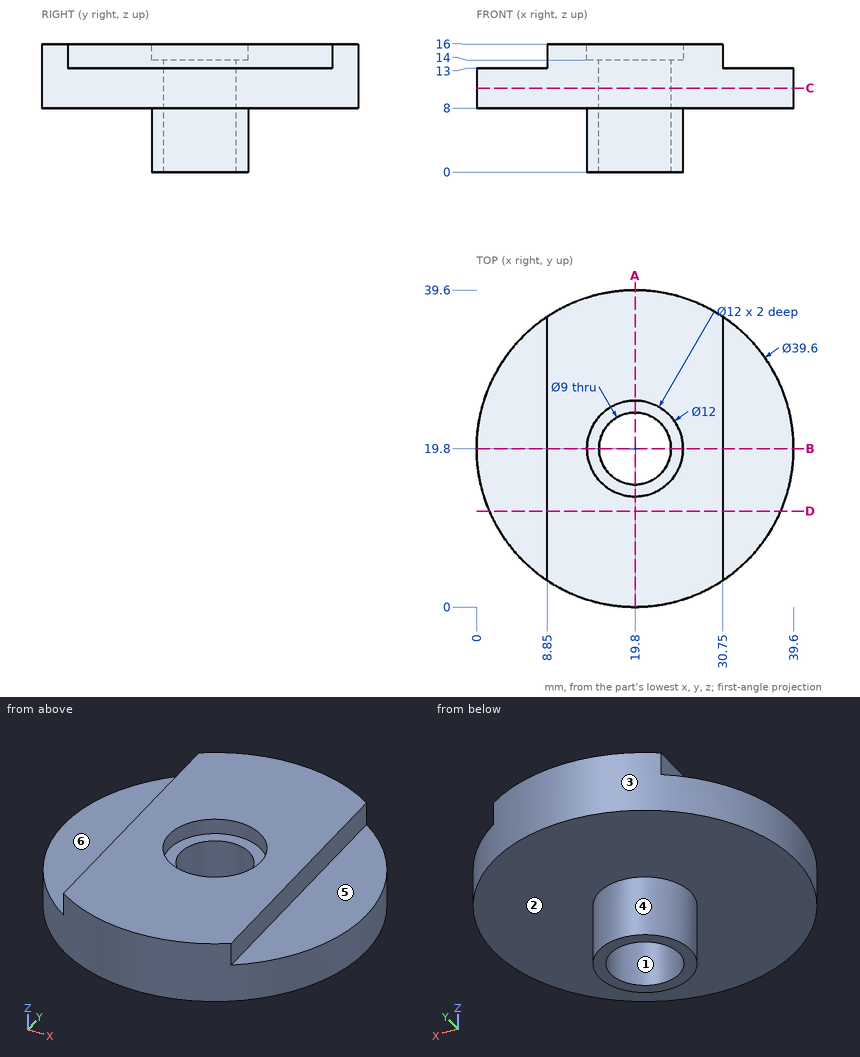
Could you check a few things on this drawing? It's one solid part, dimensions in mm from its lowest x, y, z. A direction names the side the tool comes from. Give positions to 0.01 mm unless a question says otherwise; leave off trailing zeros. Write each loop counter-clockwise with the first axis right and the second up, starting at its lowest first coordinate (ties: lowest second). Pieces come first, ordered by that corner, then holes. Notation, with made-up numbers: M 15.25,7 L 39.25,7 A8 cw 39.25,21 Z; hole C 38,37.5 d6. An arc over 180 degrees is marked long. Put each result on its own line as item: value. Start each with the question number.
Item 1: Will these pins go through, and if not, where does the flat tip stop? pin 1 (6 mm diameter, centred on y = 6, z = 7.5, fed in from -X); pin 2 (1.5 mm diameter, centred on y = 13.5, z = 14.5, fed in from -X); pin 3 (2 mm diameter, centred on y = 33, z = 10.5, fed in from +X).
Item 2: I need wall thicknesses on L1, parallel to X at y = 19.8, z = 6.75; L2, parallel to Y at x = 19.8, z = 10.75. Which ranges of each line are inside material? Lowest first, please. Write a range as from..to.
Item 3: Thinking about a two-plate mould opening in X: for the marked faces 1, 2 and 3, which applies, +X half, -X half, draft (parallel to the pull), parting line (faces both ways), or undercut?
Item 4: If we section it at D-D, the plane y = 12: Write out the boundary of the cut face in (x, z).
Item 5: If we section it at C-C, the plane z = 10.5: Write out the boundary of the cut face in (x, y), then the cut area to 3 significant figures.
Item 6: If we section it at A-A, the plane x = 19.8: Write out the boundary of the cut face in (y, z).
Item 7: If we section it at B-B, the plane y = 19.8: Write out the boundary of the cut face in (x, z), then the cut area to 3 significant figures.
Item 8: On a 3-axis mill with a long thin cutter (end or side, diameter ignored), from which of +Z, -Z, +X, -X, +Y, -Y can I reach the whole of each face in a straight line? I mean the marked faces 4, 5 and 6. Say none if no direction works.
Values:
1. pin 1: x = 3.23
1. pin 2: x = 8.85
1. pin 3: x = 35.39
2. L1: 13.8..15.3, 24.3..25.8
2. L2: 0..15.3, 24.3..39.6
3. face 1: undercut
3. face 2: draft
3. face 3: parting line
4. outline: M 1.6,8 L 38,8 L 38,13 L 30.75,13 L 30.75,16 L 8.85,16 L 8.85,13 L 1.6,13 Z
5. outline: C 19.8,19.8 d39.6; hole C 19.8,19.8 d9
5. area: 1,170 mm²
6. outline: M 0,8 L 13.8,8 L 13.8,0 L 15.3,0 L 15.3,14 L 13.8,14 L 13.8,16 L 0,16 Z; M 24.3,0 L 25.8,0 L 25.8,8 L 39.6,8 L 39.6,16 L 25.8,16 L 25.8,14 L 24.3,14 Z
7. outline: M 0,8 L 13.8,8 L 13.8,0 L 15.3,0 L 15.3,14 L 13.8,14 L 13.8,16 L 8.85,16 L 8.85,13 L 0,13 Z; M 24.3,0 L 25.8,0 L 25.8,8 L 39.6,8 L 39.6,13 L 30.75,13 L 30.75,16 L 25.8,16 L 25.8,14 L 24.3,14 Z
7. area: 210 mm²
8. face 4: -Z
8. face 5: +Z, +X, +Y, -Y
8. face 6: +Z, -X, +Y, -Y
